Part model, mm, in its own coordinate system. A direction names the side the tool comes from. Round coordinates to 2 decimals unless told otherwise and drop trailing zeros. Write each loop counter-clockwise with the first axis right and the second up, starting at its lowest first coordinate (ties: lowest second). Pieces come first, ordered by that corner, then holes. Notation, with made-up numbers: M -10,39.25 L -4,39.25 A24 cw -4,55.25 Z; hole C -19,78 d9. An arc over 180 degrees is marked long. Use a Markdown table: item, result. Add a question column.
1) Slice it at C-C on y = 3. Write the cut outline in (x, z), plus the area to 3 significant figures.
2) Wall check: probe 1 along X at (y, z) = (1.35, 10); probe 2 along Z at (x, y) = (52.5, 2.1); probe 3 along X at (y, z) = (3.95, 10). Give the ranges that are in metal, low to high.
3) Drop flat-ended pins along their axis: P1, Ø10, axis at y = 17, z = 13, coming from the +X side; P2, Ø12, axis at x = 56, z = 6.5, coming from the +Y side; P3, Ø1.5, axis at x = 20.5, z = 6, coming from the +Y side. Give the stop position or say it passes through.
4) Which spindle directions (+Z, -Z, +X, -X, +Y, -Y) get a long thin tool onto all of the face, cutting with end or side? Do faces 1 (the face through (50.8, 5, 7.6)), 2 (the face through (54.81, 2.54, 10.96)), 3 (the face through (-50.6, 5, 7.6)). Say none if no direction does.
5) Slice it at D-D on z = 4.5. Write the cut outline in (x, y).
6) Slice it at A-A on z = 10. Write the cut outline in (x, y), plus the area to 3 significant figures.
7) Slice it at B-B on x = -52.5. Write the cut outline in (y, z), plus the area to 3 significant figures.
```python
from build123d import *

# Parameters (mm, degrees)
BOSS_EXTRUDE1_DEPTH = 20
SKETCH3_R           = 2.5
CUT_EXTRUDE2_DEPTH  = 6


with BuildPart() as part:
    # Sketch1 → Boss-Extrude1 (new body)
    with BuildSketch(Plane.XY):
        with BuildLine():
            Line((-45, 0), (-40, 0))
            ThreePointArc((-40, 0), (0, 40), (40, 0))
            Line((40, 0), (45, 0))
            Line((45, 0), (60, 0))
            Line((60, 0), (60, 5))
            Line((60, 5), (44.72135955, 5))
            ThreePointArc((44.72135955, 5), (0, 45), (-44.72135955, 5))
            Line((-44.72135955, 5), (-60, 5))
            Line((-60, 5), (-60, 0))
            Line((-60, 0), (-45, 0))
        make_face()
    extrude(amount=BOSS_EXTRUDE1_DEPTH)

    # Sketch3 → Cut-Extrude2 (cut, through all)
    with BuildSketch(Plane(origin=(0, 5, 0), x_dir=(1, 0, 0), z_dir=(0, 1, 0))):
        with Locations((-52.5, -10)):
            Circle(SKETCH3_R)
        with Locations((52.5, -10)):
            Circle(SKETCH3_R)
    extrude(amount=-CUT_EXTRUDE2_DEPTH, mode=Mode.SUBTRACT)


solid = part.part
```
Entries:
| question | item | result |
|---|---|---|
| 1 | outline | M -60,0 L -39.89,0 L -39.89,20 L -60,20 Z; M 39.89,0 L 60,0 L 60,20 L 39.89,20 Z; hole C -52.5,10 d5; hole C 52.5,10 d5 |
| 1 | area | 765 mm^2 |
| 2 | probe 1 | x = -60 to -55, -50 to -39.98, 39.98 to 50, 55 to 60 |
| 2 | probe 2 | z = 0 to 7.5, 12.5 to 20 |
| 2 | probe 3 | x = -60 to -55, -50 to -39.8, 39.8 to 50, 55 to 60 |
| 3 | P1 | stops at x = 43.37 |
| 3 | P2 | stops at y = 5 |
| 3 | P3 | stops at y = 40.43 |
| 4 | face 1 | +Z, -Z, +X, +Y |
| 4 | face 2 | +Y, -Y |
| 4 | face 3 | +Z, -Z, -X, +Y |
| 5 | outline | M -60,0 L -40,0 A40 cw 40,0 L 60,0 L 60,5 L 44.72,5 A45 ccw -44.72,5 L -60,5 Z |
| 6 | outline | M -60,0 L -55,0 L -55,5 L -60,5 Z; M -50,0 L -40,0 A40 cw 40,0 L 50,0 L 50,5 L 44.72,5 A45 ccw -44.72,5 L -50,5 Z; M 55,0 L 60,0 L 60,5 L 55,5 Z |
| 6 | area | 769 mm^2 |
| 7 | outline | M 0,0 L 5,0 L 5,7.5 L 0,7.5 Z; M 0,12.5 L 5,12.5 L 5,20 L 0,20 Z |
| 7 | area | 75.0 mm^2 |
